The listing builds one solid part. Answer for the finished solid, in the listing's coordinates (mm). A direction names the side the tool comes from. Coordinates: 2 decimals unless noted, no trailing zeros. Order: outer loops, then holes, each group sorted by start corner. A loop starts at its lowest first (then second) coordinate and runs counter-clockwise, first axis right, second up.
from build123d import *

# Parameters (mm, degrees)
F1_DEPTH = 1000
F3_DEPTH = 5
F5_DEPTH = 5


with BuildPart() as f1:
    # F0 (on Front) → F1 (new body)
    with BuildSketch(Plane.XZ):
        with BuildLine():
            ThreePointArc((40, 35), (38.535534, 38.535534), (35, 40))
            Line((35, 40), (-35, 40))
            ThreePointArc((-35, 40), (-38.535534, 38.535534), (-40, 35))
            Line((-40, 35), (-40, -35))
            ThreePointArc((-40, -35), (-38.535534, -38.535534), (-35, -40))
            Line((-35, -40), (35, -40))
            ThreePointArc((35, -40), (38.535534, -38.535534), (40, -35))
            Line((40, -35), (40, 35))
        make_face()
        with BuildLine():
            ThreePointArc((-36, 35), (-35.707107, 35.707107), (-35, 36))
            Line((-35, 36), (35, 36))
            ThreePointArc((35, 36), (35.707107, 35.707107), (36, 35))
            Line((36, 35), (36, -35))
            ThreePointArc((36, -35), (35.707107, -35.707107), (35, -36))
            Line((35, -36), (-35, -36))
            ThreePointArc((-35, -36), (-35.707107, -35.707107), (-36, -35))
            Line((-36, -35), (-36, 35))
        make_face(mode=Mode.SUBTRACT)
    extrude(amount=-F1_DEPTH)

    # F2 (on face) → F3 (join)
    with BuildSketch(Plane.XY.offset(40)):
        with BuildLine():
            ThreePointArc((40, 74), (38.242641, 78.242641), (34, 80))
            Line((34, 80), (-34, 80))
            ThreePointArc((-34, 80), (-38.242641, 78.242641), (-40, 74))
            Line((-40, 74), (-40, 6))
            ThreePointArc((-40, 6), (-38.242641, 1.757359), (-34, 0))
            Line((-34, 0), (34, 0))
            ThreePointArc((34, 0), (38.242641, 1.757359), (40, 6))
            Line((40, 6), (40, 74))
        make_face()
        with BuildLine():
            ThreePointArc((34, 76), (35.414214, 75.414214), (36, 74))
            Line((36, 74), (36, 6))
            ThreePointArc((36, 6), (35.414214, 4.585786), (34, 4))
            Line((34, 4), (-34, 4))
            ThreePointArc((-34, 4), (-35.414214, 4.585786), (-36, 6))
            Line((-36, 6), (-36, 74))
            ThreePointArc((-36, 74), (-35.414214, 75.414214), (-34, 76))
            Line((-34, 76), (34, 76))
        make_face(mode=Mode.SUBTRACT)
    extrude(amount=F3_DEPTH)

    # F4 (on face) → F5 (join)
    with BuildSketch(Plane.XY.offset(40)):
        with BuildLine():
            ThreePointArc((40, 994), (38.242641, 998.242641), (34, 1000))
            Line((34, 1000), (-34, 1000))
            ThreePointArc((-34, 1000), (-38.242641, 998.242641), (-40, 994))
            Line((-40, 994), (-40, 926))
            ThreePointArc((-40, 926), (-38.242641, 921.757359), (-34, 920))
            Line((-34, 920), (34, 920))
            ThreePointArc((34, 920), (38.242641, 921.757359), (40, 926))
            Line((40, 926), (40, 994))
        make_face()
        with BuildLine():
            ThreePointArc((34, 996), (35.414214, 995.414214), (36, 994))
            Line((36, 994), (36, 926))
            ThreePointArc((36, 926), (35.414214, 924.585786), (34, 924))
            Line((34, 924), (-34, 924))
            ThreePointArc((-34, 924), (-35.414214, 924.585786), (-36, 926))
            Line((-36, 926), (-36, 994))
            ThreePointArc((-36, 994), (-35.414214, 995.414214), (-34, 996))
            Line((-34, 996), (34, 996))
        make_face(mode=Mode.SUBTRACT)
    extrude(amount=F5_DEPTH)


solid = f1.part
(1) Find the intervals of material crossed by probe 1 along Y at (x, z) = (-27.5, 41.5); probe 2 along Z at (x, y) = (12, 108.5); probe 3 along Z at (x, y) = (35.5, 937), in increasing order.
(2) The mould has two halves that part along Z. Classify faces 1 (the flat face through (0, 493, -36)), 2 (the flat face through (0, 493, -40)), 3 (the flat face through (0, 959, 40)): pulls with the +Z half, pulls with the -Z half, needs draft (parallel to the pull), parting line crosses it, or undercut.
(3) Find section B-B on z = -5. Determine the outline of the cut face in (x, y).
(4) Given pin 1 Ø1 at (x, y) = (11, 697) entering from +Z; pin 2 Ø2.5 at (x, y) = (37, 53.5) entering from -Z, each flat-ended and moving along its own axis, determine where each tip first touches the part or whether it passes through.
(5) Find section C-C on y = 205. Determine the outline of the cut face in (x, z).
(6) Find section A-A on x = -7.5. Determine the outline of the cut face in (y, z).
(7) A tool of negligible diameter and unlimited length cuts with its end or side. For faces 4 (the flat face through (0, 39, 40)), 5 (the flat face through (0, 494, 40)), 6 (the flat face through (36, 493, 0)), from which of +Z, -Z, +X, -X, +Y, -Y can it reach the whole face along a straight path? Write none if from no direction.
Resolved:
1. probe 1: y = 0 to 4, 76 to 80, 920 to 924, 996 to 1000
1. probe 2: z = -40 to -36, 36 to 40
1. probe 3: z = -39.97 to -35.87, 35.87 to 39.97
2. face 1: undercut
2. face 2: pulls with the -Z half
2. face 3: pulls with the +Z half
3. outline: (-40, 0) - (-36, 0) - (-36, 1000) - (-40, 1000) - close; (36, 0) - (40, 0) - (40, 1000) - (36, 1000) - close
4. pin 1: stops at z = 40
4. pin 2: stops at z = -39.94
5. outline: (-40, -35) arc R5 ccw to (-35, -40) - (35, -40) arc R5 ccw to (40, -35) - (40, 35) arc R5 ccw to (35, 40) - (-35, 40) arc R5 ccw to (-40, 35) - close; hole (-36, -35) arc R1 ccw to (-35, -36) - (35, -36) arc R1 ccw to (36, -35) - (36, 35) arc R1 ccw to (35, 36) - (-35, 36) arc R1 ccw to (-36, 35) - close
6. outline: (0, -40) - (1000, -40) - (1000, -36) - (0, -36) - close; (0, 36) - (1000, 36) - (1000, 45) - (996, 45) - (996, 40) - (924, 40) - (924, 45) - (920, 45) - (920, 40) - (80, 40) - (80, 45) - (76, 45) - (76, 40) - (4, 40) - (4, 45) - (0, 45) - close
7. face 4: +Z
7. face 5: +Z, +X, -X
7. face 6: +Y, -Y
